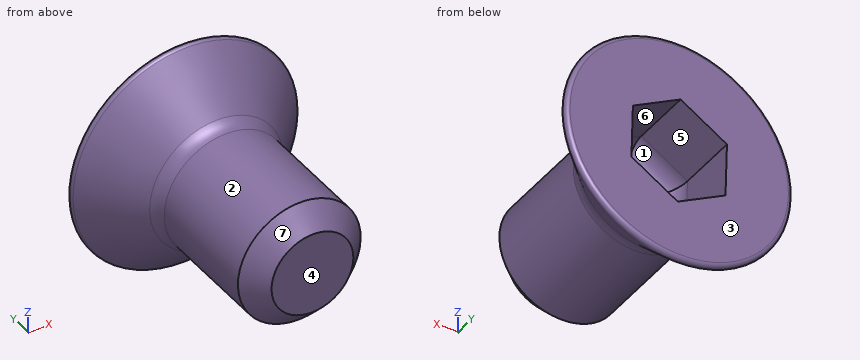
Autodesk Inventor part; units mm, degrees
ref_plane "YZ Plane" through (0, 0, 0) normal (1, 0, 0) x (0, 1, 0)
ref_plane "XZ Plane" through (0, 0, 0) normal (0, 1, 0) x (-1, 0, 0)
ref_plane "XY Plane" through (0, 0, 0) normal (0, 0, 1) x (1, 0, 0)
sketch "Szkic2" plane through (0, 0, 0) normal (1, 0, 0) x (0, 1, 0)
  line L0 (0, -2.9) -> (0, 2.9)
  line L1 (-1.5, -1.5) -> (-1.5, 1.5)
  line L2 (-1.5, -1.5) -> (0, -2.9)
  line L3 (-1.5, 1.5) -> (0, 2.9)
  line L4 (0, 0) -> (-5, 0)
  line L5 (-5, 0) -> (-5, -1.5)
  line L6 (-5, -1.5) -> (-1.5, -1.5)
  dimension "d0" = 5.8
  dimension "d2" = 3
  dimension "d3" = 1.5
  dimension "d4" = 5
  dimension "d5" = 1.5
revolve "Obrót1" add sketch "Szkic2" angle 360 about axis through (0, 0, 0) along (0, -1, 0) contours L2 L1 L4 L0 | L6 L5 L4 L1
sketch "Szkic3" plane through (0, 0, 0) normal (0, 1, 0) x (1, 0, 0)
  line L0 (-1.1673, -0.633) -> (-1.1318, 0.6945)
  line L1 (-1.1318, 0.6945) -> (0.0355, 1.3274)
  line L2 (0.0355, 1.3274) -> (1.1673, 0.633)
  line L3 (1.1673, 0.633) -> (1.1318, -0.6945)
  line L4 (1.1318, -0.6945) -> (-0.0355, -1.3274)
  line L5 (-0.0355, -1.3274) -> (-1.1673, -0.633)
  point P0 (0, 0)
  point P1 (0, 0)
  dimension "d7" = 2.3
extrude "Wyciągnięcie proste1" cut sketch "Szkic3" against normal blind 2
fillet "Zaokrąglenie1" radius 0.5 6 edges at (-1.1496, -2, -0.0308) (-0.6014, -2, 0.9802) (-0.5482, -2, -1.011) (0.6014, -2, -0.9802) (0.5482, -2, 1.011) (1.1496, -2, 0.0308)
fillet "Zaokrąglenie2" radius 0.5 1 edges at (0, -1.5, 1.5)
fillet "Zaokrąglenie3" radius 0.1 1 edges at (0, 0, 2.9)
thread "Gwint1"
chamfer "Faza1" distance 0.5 angle 45 1 edges at (0, -5, 1.5)
properties part number "Screw M3 5mm flat head"
Here's how the part is built. I have some questions about the finished solid (model axes, mm). Face numbers are marked on the shaded views. A direction names the side the tool comes from. Give positions to 0.01 mm unless a question says otherwise; leave off trailing zeros. Order: outer loops, then holes, each group sorted by start corner. A loop starts at its lowest first (then second) coordinate and runs counter-clockwise, first axis right, second up. Notation, with made-up numbers: (44.5, -18.5) -> (73.5, -18.5) arc R33 cw to (73.5, 13.5) -> close; hole circle Ø1 at (68.25, 83.5). An arc over 180 degrees is marked (long way). One line per item, written item: value. Start each with the question number.
1. Imagine slicing it at B-B, the plane y = -0.4. List the corners of the cut face in (x, z) for me.
2. Will these pins go through, and if not, where does the flat tip stop? pin 1 Ø1 at (y, z) = (-2, -1) entering from -X; pin 2 Ø1 at (x, z) = (1, -1.5) entering from -Y.
3. I need wall thicknesses on probe 1 along Y at (x, z) = (2.1, -0.65); probe 2 along Y at (x, z) = (0, -0.6); probe 3 along X at (y, z) = (-0.75, -0.75). Which ranges of each line are inside material? Lowest first, please. Write a range as from..to.
4. Imagine slicing it at A-A, the plane y = -1.8. List the corners of the cut face in (x, z) for me, plus the area to 3 significant figures.
5. For the marked faces 1, 2 and 3, which set-ups out of +Z, -Z, +X, -X, +Y, -Y let a thin tool reach every point of the face, with its end or its side?
6. We'd pull the mould along Z, two halves only. Please class the marked faces 4, 5, 6 and 7: released by +Z, released by -Z, zero draft, split by the parting line, or undercut.
7. Imagine slicing it at C-C, the plane y = -2.55. List the corners of the cut face in (x, z) for me, plus the area to 3 significant figures.
Values follow:
1. outline: circle Ø5.05 at (0, 0); hole (-1.17, 0.63) -> (-1.13, -0.69) -> (0.04, -1.33) -> (1.17, -0.63) -> (1.13, 0.69) -> (-0.04, 1.33) -> close
2. pin 1: stops at x = -1.41
2. pin 2: stops at y = -4.7
3. probe 1: y = -0.75..0
3. probe 2: y = -5..-2
3. probe 3: x = -2.07..-1.03, 0.98..2.07
4. outline: circle Ø3 at (0, 0); hole (-1.07, 0.58) -> (-1.03, -0.63) -> (0.03, -1.21) -> (1.07, -0.58) -> (1.03, 0.63) -> (-0.03, 1.21) -> close
4. area: 3.25 mm2
5. face 1: +Y
5. face 2: -Y
5. face 3: +Z, -Z, +X, -X, +Y
6. face 4: zero draft
6. face 5: undercut
6. face 6: undercut
6. face 7: split by the parting line
7. outline: circle Ø3 at (0, 0)
7. area: 7.07 mm2
